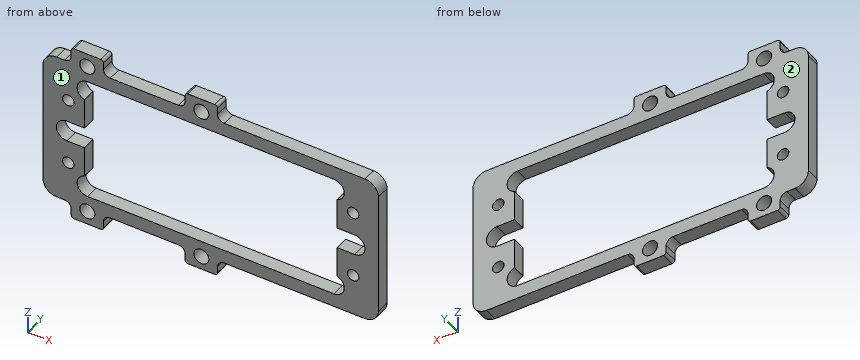
from build123d import *

# Parameters (mm, degrees)
SKETCH1_R           = 1.35255
SKETCH1_R_2         = 1.778
BOSS_EXTRUDE1_DEPTH = 3.175


with BuildPart() as part:
    # Sketch1 → Boss-Extrude1 (new body)
    with BuildSketch(Plane.XZ):
        with BuildLine():
            Line((-6.02234, -19.2405), (-6.02234, -20.828))
            ThreePointArc((-6.02234, -20.828), (-5.836352806, -21.277012806), (-5.38734, -21.463))
            Line((-5.38734, -21.463), (0.96266, -21.463))
            ThreePointArc((0.96266, -21.463), (1.411672806, -21.277012806), (1.59766, -20.828))
            Line((1.59766, -20.828), (1.59766, -19.2405))
            ThreePointArc((1.59766, -19.2405), (2.062627985, -18.117967985), (3.18516, -17.653))
            Line((3.18516, -17.653), (36.43122, -17.653))
            ThreePointArc((36.43122, -17.653), (38.688856389, -16.717856389), (39.624, -14.46022))
            Line((39.624, -14.46022), (39.624, 14.46022))
            ThreePointArc((39.624, 14.46022), (38.688856389, 16.717856389), (36.43122, 17.653))
            Line((36.43122, 17.653), (3.18516, 17.653))
            ThreePointArc((3.18516, 17.653), (2.062627985, 18.117967985), (1.59766, 19.2405))
            Line((1.59766, 19.2405), (1.59766, 20.828))
            ThreePointArc((1.59766, 20.828), (1.411672806, 21.277012806), (0.96266, 21.463))
            Line((0.96266, 21.463), (-5.38734, 21.463))
            ThreePointArc((-5.38734, 21.463), (-5.836352806, 21.277012806), (-6.02234, 20.828))
            Line((-6.02234, 20.828), (-6.02234, 19.2405))
            ThreePointArc((-6.02234, 19.2405), (-6.487307985, 18.117967985), (-7.60984, 17.653))
            Line((-7.60984, 17.653), (-23.755604, 17.653))
            ThreePointArc((-23.755604, 17.653), (-24.878136015, 18.117967985), (-25.343104, 19.2405))
            Line((-25.343104, 19.2405), (-25.343104, 20.828))
            ThreePointArc((-25.343104, 20.828), (-25.529091194, 21.277012806), (-25.978104, 21.463))
            Line((-25.978104, 21.463), (-32.328104, 21.463))
            ThreePointArc((-32.328104, 21.463), (-32.777116806, 21.277012806), (-32.963104, 20.828))
            Line((-32.963104, 20.828), (-32.963104, 19.2405))
            ThreePointArc((-32.963104, 19.2405), (-33.428071985, 18.117967985), (-34.550604, 17.653))
            Line((-34.550604, 17.653), (-36.43122, 17.653))
            ThreePointArc((-36.43122, 17.653), (-38.688856389, 16.717856389), (-39.624, 14.46022))
            Line((-39.624, 14.46022), (-39.624, -14.46022))
            ThreePointArc((-39.624, -14.46022), (-38.688856389, -16.717856389), (-36.43122, -17.653))
            Line((-36.43122, -17.653), (-34.550604, -17.653))
            ThreePointArc((-34.550604, -17.653), (-33.428071985, -18.117967985), (-32.963104, -19.2405))
            Line((-32.963104, -19.2405), (-32.963104, -20.828))
            ThreePointArc((-32.963104, -20.828), (-32.777116806, -21.277012806), (-32.328104, -21.463))
            Line((-32.328104, -21.463), (-25.978104, -21.463))
            ThreePointArc((-25.978104, -21.463), (-25.529091194, -21.277012806), (-25.343104, -20.828))
            Line((-25.343104, -20.828), (-25.343104, -19.2405))
            ThreePointArc((-25.343104, -19.2405), (-24.878136015, -18.117967985), (-23.755604, -17.653))
            Line((-23.755604, -17.653), (-7.60984, -17.653))
            ThreePointArc((-7.60984, -17.653), (-6.487307985, -18.117967985), (-6.02234, -19.2405))
        make_face()
        with Locations((33.655, -7.874)):
            Circle(SKETCH1_R, mode=Mode.SUBTRACT)
        with Locations((-33.655, 7.874)):
            Circle(SKETCH1_R, mode=Mode.SUBTRACT)
        with Locations((-33.655, -7.874)):
            Circle(SKETCH1_R, mode=Mode.SUBTRACT)
        with Locations((-2.21234, 18.288)):
            Circle(SKETCH1_R_2, mode=Mode.SUBTRACT)
        with Locations((-29.153104, -18.288)):
            Circle(SKETCH1_R_2, mode=Mode.SUBTRACT)
        with Locations((-2.21234, -18.288)):
            Circle(SKETCH1_R_2, mode=Mode.SUBTRACT)
        with Locations((-29.153104, 18.288)):
            Circle(SKETCH1_R_2, mode=Mode.SUBTRACT)
        with Locations((33.655, 7.874)):
            Circle(SKETCH1_R, mode=Mode.SUBTRACT)
        with BuildLine():
            Line((-33.9725, 2.4765), (-29.845, 2.4765))
            Line((-29.845, 2.4765), (-29.845, 9.645968035))
            ThreePointArc((-29.845, 9.645968035), (-31.52653105, 12.388525412), (-29.08046, 14.478))
            Line((-29.08046, 14.478), (29.08046, 14.478))
            ThreePointArc((29.08046, 14.478), (31.52653105, 12.388525412), (29.845, 9.645968035))
            Line((29.845, 9.645968035), (29.845, 2.4765))
            Line((29.845, 2.4765), (33.9725, 2.4765))
            ThreePointArc((33.9725, 2.4765), (36.449, 0), (33.9725, -2.4765))
            Line((33.9725, -2.4765), (29.845, -2.4765))
            Line((29.845, -2.4765), (29.845, -9.645968035))
            ThreePointArc((29.845, -9.645968035), (31.52653105, -12.388525412), (29.08046, -14.478))
            Line((29.08046, -14.478), (-29.08046, -14.478))
            ThreePointArc((-29.08046, -14.478), (-31.52653105, -12.388525412), (-29.845, -9.645968035))
            Line((-29.845, -9.645968035), (-29.845, -2.4765))
            Line((-29.845, -2.4765), (-33.9725, -2.4765))
            ThreePointArc((-33.9725, -2.4765), (-36.449, 0), (-33.9725, 2.4765))
        make_face(mode=Mode.SUBTRACT)
    extrude(amount=-BOSS_EXTRUDE1_DEPTH)


solid = part.part
Here's how the part is built. I have some questions about the finished solid (model axes, mm). Face numbers are marked on the shaded views. Coordinates: 2 decimals unless noted, no trailing zeros. Write each loop counter-clockwise with the first axis right and the second up, starting at its lowest first coordinate (ties: lowest second). Pieces come first, ordered by that corner, then holes.
Item 1: I want a section at C-C on y = 2.65. Count the separate pieces of the cut face and the enclosed holes in it, and give its area (3 significant figures).
Item 2: If we mould it in two halves opening along Y, with no side actions, what happens to the marked faces 1 and 2? For each: +Y half, -Y half, draft (parallel to the pull), parting line (faces both ways), or undercut.
Item 3: If I drill on line 1 (X direction, y = 1.9, z = 6) (3 decimals); line 2 (Z direction, x = -10.5, y = 0.4); line 3 (Z direction, x = 0.5, y = 1.1), over which ranges is the centre line in solid material (lowest first)?
Item 4: I want a section at B-B on z = 0. Write out the boundary of the cut face in (x, y) (3 decimals).
Item 5: I want a section at A-A on x = 25. Write out the boundary of the cut face in (y, z) (3 decimals), and give its area (3 significant figures).
Item 6: Will these pins go through, and if not, where does the flat tip stop? pin 1 (1 mm diameter, centred on x = 31.5, y = 2, fed in from +Z); pin 2 (0.9 mm diameter, centred on x = -35.5, y = 2, fed in from -Z); pin 3 (1.7 mm diameter, centred on y = 2.5, z = 20, fed in from +X).
Findings below:
1. separate pieces: 1
1. enclosed holes: 9
1. area: 1,030 mm2
2. face 1: -Y half
2. face 2: +Y half
3. line 1: x = -39.624 to -29.845, 29.845 to 39.624
3. line 2: z = -17.65 to -14.48, 14.48 to 17.65
3. line 3: z = -21.46 to -14.48, 14.48 to 21.46
4. outline: (-39.624, 0) - (-36.449, 0) - (-36.449, 3.175) - (-39.624, 3.175) - close; (36.449, 0) - (39.624, 0) - (39.624, 3.175) - (36.449, 3.175) - close
5. outline: (0, -17.653) - (3.175, -17.653) - (3.175, -14.478) - (0, -14.478) - close; (0, 14.478) - (3.175, 14.478) - (3.175, 17.653) - (0, 17.653) - close
5. area: 20.2 mm2
6. pin 1: stops at z = 17.65
6. pin 2: stops at z = -17.65
6. pin 3: stops at x = 1.6
